```python
from build123d import *

# Parameters (mm, degrees)
SKETCH_1_R          = 13.5
SKETCH_1_R_2        = 5
EXTRUDE_1_DEPTH     = 4
SKETCH_2_R          = 1.45
CUT_EXTRUDE_1_DEPTH = 90.899944383
SKETCH_4_R          = 1.45
CUT_EXTRUDE_3_DEPTH = 90.899944383
FILLET_4_R          = 5
CUT_EXTRUDE_4_DEPTH = 90.899944383
FILLET_5_R          = 2


with BuildPart() as part:
    # 草图1 → 凸台-拉伸1 (new body)
    with BuildSketch(Plane.XY):
        with BuildLine():
            Line((-55, 0), (-55, -15))
            ThreePointArc((-55, -15), (-20.693136595, -25.465682976), (15, -29))
            ThreePointArc((15, -29), (17.07003357, -28.900115911), (19.120833333, -28.601391723))
            Line((19.120833333, -28.601391723), (76.916666667, -17.314600801))
            ThreePointArc((76.916666667, -17.314600801), (85, -7.5), (76.916666667, 2.314600801))
            Line((76.916666667, 2.314600801), (19.120833333, 13.601391723))
            ThreePointArc((19.120833333, 13.601391723), (17.07003357, 13.900115911), (15, 14))
            ThreePointArc((15, 14), (-20.693136595, 10.465682976), (-55, 0))
        make_face()
        with Locations((15, -7.5)):
            Circle(SKETCH_1_R, mode=Mode.SUBTRACT)
        with Locations((75, -7.5)):
            Circle(SKETCH_1_R_2, mode=Mode.SUBTRACT)
    extrude(amount=EXTRUDE_1_DEPTH)

    # 草图2 → 切除-拉伸1 (cut, through all)
    with BuildSketch(Plane.XY.offset(4)):
        with Locations((-45, -7.5)):
            Circle(SKETCH_2_R)
        with Locations((-35, -7.5)):
            Circle(SKETCH_2_R)
        with Locations((-25, -7.5)):
            Circle(SKETCH_2_R)
    extrude(amount=-CUT_EXTRUDE_1_DEPTH, mode=Mode.SUBTRACT)

    # 草图4 → 切除-拉伸3 (cut, through all)
    with BuildSketch(Plane(origin=(0, 0, 0), x_dir=(-1, 0, 0), z_dir=(0, 0, -1))):
        with Locations((-59, -7.117300414)):
            Circle(SKETCH_4_R)
        with Locations((-48.359904235, -17.69030198)):
            Circle(SKETCH_4_R)
    extrude(amount=-CUT_EXTRUDE_3_DEPTH, mode=Mode.SUBTRACT)

    # 圆角4
    fillet_4_edges = [part.edges().sort_by_distance(p)[0] for p in [
        (-55, -15, 2),
        (-55, 0, 2),
    ]]
    fillet(fillet_4_edges, radius=FILLET_4_R)

    # 草图5 → 切除-拉伸4 (cut, through all)
    with BuildSketch(Plane.XY.offset(4)):
        with BuildLine():
            Line((-37.662714363, -0.06358788), (-5.309418997, -0.06358788))
            ThreePointArc((-5.309418997, -0.06358788), (-3.415372639, 3.842256204), (-0.779510023, 7.291206463))
            ThreePointArc((-0.779510023, 7.291206463), (-19.418131409, 4.60183148), (-37.662714363, -0.06358788))
        make_face()
        with BuildLine():
            Line((-37.271815743, -15.058493623), (-5.264301107, -15.058493623))
            ThreePointArc((-5.264301107, -15.058493623), (-3.381161932, -18.897614279), (-0.779510023, -22.291206463))
            ThreePointArc((-0.779510023, -22.291206463), (-19.217302179, -19.641756918), (-37.271815743, -15.058493623))
        make_face()
        with BuildLine():
            Line((31.138502072, 5.141153068), (58.805420584, -0.261844115))
            Line((58.805420584, -0.261844115), (41.950078957, -17.010899515))
            Line((41.950078957, -17.010899515), (32.001874449, -18.953657286))
            ThreePointArc((32.001874449, -18.953657286), (35.486852137, -6.765909049), (31.138502072, 5.141153068))
        make_face()
    extrude(amount=-CUT_EXTRUDE_4_DEPTH, mode=Mode.SUBTRACT)

    # 圆角5
    fillet_5_edges = [part.edges().sort_by_distance(p)[0] for p in [
        (32.001874449, -18.953657286, 2),
        (31.138502072, 5.141153068, 2),
        (58.805420584, -0.261844115, 2),
        (41.950078957, -17.010899515, 2),
        (-37.662714363, -0.06358788, 2),
        (-0.779510023, 7.291206463, 2),
        (-5.309418997, -0.06358788, 2),
        (-0.779510023, -22.291206463, 2),
        (-37.271815743, -15.058493623, 2),
        (-5.264301107, -15.058493623, 2),
    ]]
    fillet(fillet_5_edges, radius=FILLET_5_R)


solid = part.part
```
Verification items for the finished model (mm, model axes). A direction names the side the tool comes from. Coordinates: 2 decimals unless noted, no trailing zeros. Loops run counter-clockwise (first coordinate to the right, second up) from the corner with the lowest first, then second, coordinate; pieces in that order, holes last. Notation, with made-up numbers: (50.5, 16.25) -> (77.5, 16.25) arc R23 cw to (77.5, 28.25) -> close; hole circle Ø1 at (73.25, -5.5). An arc over 180 degrees is marked (long way). Answer in a Markdown table with one row per item.
1) Section check A-A (x = 59). Record the cut outline in (y, z).
The answers:
| item | result |
|---|---|
| outline | (-20.81, 0) -> (-8.57, 0) -> (-8.57, 4) -> (-20.81, 4) -> close; (-5.67, 0) -> (5.81, 0) -> (5.81, 4) -> (-5.67, 4) -> close |
2) Access from +Z, -Z, +X, -X, +Y, -Y to the whole of each face (thin tool, end or side, straight path). Record for faces 1 (the face through (56.643, -0.95, 1.972)), 2 (the face through (-54.16, -14.41, 2.03)).
The answers:
| item | result |
|---|---|
| face 1 | +Z, -Z |
| face 2 | +Z, -Z, -X, -Y |
3) Depth check by flat-ended pin: P1, Ø9, axis at x = 75, y = -7.5, coming from the -Z side; P2, Ø2, axis at x = -13.5, z = 1.5, coming from the -Y side. Enter the tip coordinate at first touch or a pass-through.
The answers:
| item | result |
|---|---|
| P1 | passes through |
| P2 | stops at y = -26.91 |
4) Section check B-B (x = 75). Record the cut outline in (y, z), and give its area (3 significant figures).
The answers:
| item | result |
|---|---|
| outline | (-17.69, 0) -> (-12.5, 0) -> (-12.5, 4) -> (-17.69, 4) -> close; (-2.5, 0) -> (2.69, 0) -> (2.69, 4) -> (-2.5, 4) -> close |
| area | 41.5 mm2 |
5) Draft check along Y on faces 3 (the face through (45.23, 2.39, 2.03)), 4 (the face through (-24.37, 1.68, 1.97)), 5 (the face through (-55, -7, 2)), 6 (the face through (-54.16, -0.59, 2.03)). Enter one of: released by +Y, released by -Y, zero draft, split by the parting line, or undercut.
The answers:
| item | result |
|---|---|
| face 3 | undercut |
| face 4 | undercut |
| face 5 | zero draft |
| face 6 | released by +Y |
6) Section check D-D (y = -24). Record the cut outline in (x, z), and give its area (3 significant figures).
The answers:
| item | result |
|---|---|
| outline | (-27.37, 0) -> (42.68, 0) -> (42.68, 4) -> (-27.37, 4) -> close |
| area | 280 mm2 |
7) Section check C-C (z = 2.55). Give the number of separate pieces and of enclosed holes in the cut face, and give its area (3 significant figures).
The answers:
| item | result |
|---|---|
| separate pieces | 1 |
| enclosed holes | 10 |
| area | 3,220 mm2 |
8) Scan lines: line 1 along X through (y, z) = (-12, 2); line 2 along X through (y, z) = (-3.5, 3.05); line 3 along Y through (x, z) = (-14.5, 3.25). Record each from-to range of solid material in increasing order. Write a range as from..to.
The answers:
| item | result |
|---|---|
| line 1 | x = -54.99..2.27, 27.73..35, 46.99..72.82, 77.18..83.93 |
| line 2 | x = -55..2.11, 27.89..35.11, 55.55..72, 78..84.17 |
| line 3 | y = -26.59..-20.51, -15.06..-0.06, 5.51..11.59 |
